Read the model definition and answer for the solid it produces. Units are mm, in the model's axes. Face numbers are marked on the shaded views. A direction names the side the tool comes from. Coordinates: 2 decimals unless noted, no trailing zeros. Loops run counter-clockwise (first coordinate to the right, second up) from the corner with the lowest first, then second, coordinate; pieces in that order, holes last.
from build123d import *

# Parameters (mm, degrees)
SKETCH1_W                                        = 30
SKETCH1_H                                        = 42.7
SKETCH1_R                                        = 3.175
SKETCH1_W_2                                      = 20
SKETCH1_H_2                                      = 8.5
BOSS_EXTRUDE1_DEPTH                              = 12.7
CSK_FOR_1_4_FLAT_HEAD_MACHINE_SCREW1_D           = 7.14248
CSK_FOR_1_4_FLAT_HEAD_MACHINE_SCREW1_CSINK_D     = 12.8778
CSK_FOR_1_4_FLAT_HEAD_MACHINE_SCREW1_CSINK_ANGLE = 82
SKETCH3_W                                        = 8
SKETCH3_H                                        = 12.8
CUT_EXTRUDE1_DEPTH                               = 2.35
SKETCH4_W                                        = 4.75
SKETCH4_H                                        = 8.5
BOSS_EXTRUDE2_DEPTH                              = 1.63


with BuildPart() as part:
    # Sketch1 → Boss-Extrude1 (new body)
    with BuildSketch(Plane(origin=(0, 0, 0), x_dir=(0, 0, -1), z_dir=(1, 0, 0))):
        with Locations((15, -12.85)):
            Rectangle(SKETCH1_W, SKETCH1_H)
        with Locations((12.7, -21.5)):
            Circle(SKETCH1_R, mode=Mode.SUBTRACT)
        with Locations((-10, 4.25)):
            Rectangle(SKETCH1_W_2, SKETCH1_H_2)
    extrude(amount=BOSS_EXTRUDE1_DEPTH)

    # CSK for 1/4 Flat Head Machine Screw1 (through all)
    with Locations(Plane(origin=(12.7, -21.5, -12.7), x_dir=(0, 0, 1), z_dir=(1, 0, 0))):
        with Locations((0, 0)):
            CounterSinkHole(CSK_FOR_1_4_FLAT_HEAD_MACHINE_SCREW1_D / 2, CSK_FOR_1_4_FLAT_HEAD_MACHINE_SCREW1_CSINK_D / 2, counter_sink_angle=CSK_FOR_1_4_FLAT_HEAD_MACHINE_SCREW1_CSINK_ANGLE)

    # Sketch3 → Cut-Extrude1 (cut)
    with BuildSketch(Plane.ZY):
        with Locations((-4, -6.4)):
            Rectangle(SKETCH3_W, SKETCH3_H)
    extrude(amount=-CUT_EXTRUDE1_DEPTH, mode=Mode.SUBTRACT)

    # Sketch4 → Boss-Extrude2 (add)
    with BuildSketch(Plane.ZY):
        with Locations((5.995, 4.25)):
            Rectangle(SKETCH4_W, SKETCH4_H)
    extrude(amount=BOSS_EXTRUDE2_DEPTH)


solid = part.part
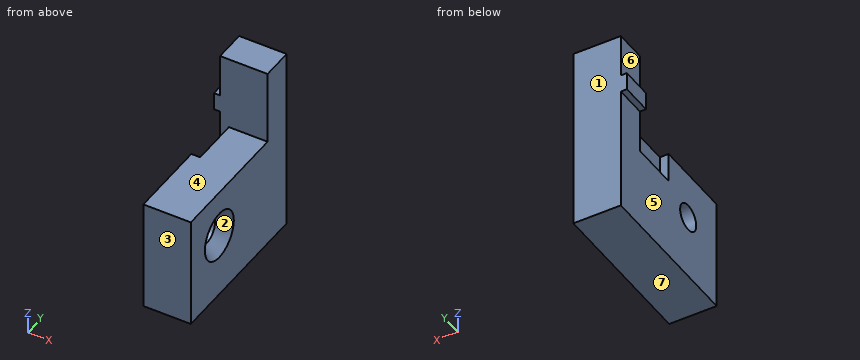
Item 1: A cutting plane is placed at D-D on y = -1.5. Determine the outline of the cut face in (x, z).
Numbers:
outline: (0, -30) - (12.7, -30) - (12.7, 0) - (2.35, 0) - (2.35, -8) - (0, -8) - close
Item 2: Find the intervals of material crossed by line 1 along Y through (x, z) = (6.75, -12.7); line 2 along Z through (x, y) = (6, -21.5); line 3 along X through (y, z) = (-22.5, -23), in increasing order.
Numbers:
line 1: y = -34.2 to -25.07, -17.93 to 8.5
line 2: z = -30 to -16.27, -9.13 to 0
line 3: x = 0 to 12.7
Item 3: A cutting plane is placed at C-C on x = 6. Determine the outline of the cut face in (y, z).
Numbers:
outline: (-34.2, -30) - (8.5, -30) - (8.5, 20) - (0, 20) - (0, 0) - (-34.2, 0) - close; hole circle Ø7.14 at (-21.5, -12.7)
Item 4: A cutting plane is placed at A-A on z = -12.7. Determine the outline of the cut face in (x, y), then the cut area to 3 significant figures.
Numbers:
outline: (0, -34.2) - (12.7, -34.2) - (12.7, -27.94) - (9.4, -25.07) - (0, -25.07) - close; (0, -17.93) - (9.4, -17.93) - (12.7, -15.06) - (12.7, 8.5) - (0, 8.5) - close
area: 442 mm2
Item 5: Determine the mould class of the marked faces 1, 2, 3 and 4 for opening direction Y: released by +Y, released by -Y, zero draft, split by the parting line, or undercut.
Numbers:
face 1: released by +Y
face 2: undercut
face 3: released by -Y
face 4: zero draft
Item 6: A cutting plane is placed at B-B on y = -21.5. Determine the outline of the cut face in (x, z), then the cut area to 3 significant figures.
Numbers:
outline: (0, -30) - (12.7, -30) - (12.7, -19.14) - (9.4, -16.27) - (0, -16.27) - close; (0, -9.13) - (9.4, -9.13) - (12.7, -6.26) - (12.7, 0) - (0, 0) - close
area: 281 mm2
Item 7: Which of the six approach directions +Z, -Z, +X, -X, +Y, -Y give full straight-line access (tool end or side, diameter ignored) to the marked faces 5, 6 and 7?
Numbers:
face 5: -Z, -X, +Y, -Y
face 6: +Z, -X, +Y, -Y
face 7: -Z, +X, -X, +Y, -Y
Item 8: Given pin 1 (1.3 mm diameter, centred on x = -1, y = 5, fed in from -Z); pin 2 (2 mm diameter, centred on y = -7.5, z = -20.5, fed in from -X); pin 3 (1.9 mm diameter, centred on x = 1, y = -6, fed in from +Z), each flat-ended and moving along its own axis, determine where each tip first touches the part or whether it passes through.
Numbers:
pin 1: stops at z = 3.62
pin 2: stops at x = 0
pin 3: stops at z = -8
